The listing builds one solid part. Answer for the finished solid, in the listing's coordinates (mm). Face numbers are marked on the shaded views. A direction names the side the tool comes from. Coordinates: 2 decimals unless noted, no trailing zeros. Loops run counter-clockwise (first coordinate to the right, second up) from the corner with the lowest first, then second, coordinate; pieces in that order, holes last. Notation, with made-up numbers: (-24, -37) - (18, -37) arc R25 ccw to (18, -6) - close; hole circle Ø5 at (75.25, -13.5). An arc over 180 degrees is marked (long way). Return JSON: item names as keys, results as strings. Group by question number.
1. Each of these flat-tipped pins is pushed along its axis until it touches: P1, Ø8, axis at y = -22.5, z = 14.5, coming from the -X side; P2, Ø1, axis at y = -4.5, z = 14, coming from the +X side; P3, Ø5, axis at y = -8.5, z = 7, coming from the +X side. Where does it stop, or does it pass through?
2. Section C-C (y = -10) is taken. Write down the section's boundary in (x, z), and give its area (3 significant figures).
3. Section B-B (y = -2.5) is taken. Write down the section's boundary in (x, z), and give its area (3 significant figures).
4. Which of the six approach directions +Z, -Z, +X, -X, +Y, -Y give full straight-line access (tool end or side, diameter ignored) to the marked faces 1 and 2?
5. Find the intervals of material crossed by line 1 along X through (y, z) = (-16.5, -0.5); line 2 along X through (y, z) = (-2, 11.5); line 3 along X through (y, z) = (-13.75, 18), in increasing order.
6. The mould has two halves that part along X. Classify the marked faces 3, 4, 5 and 6: pulls with the +X half, pulls with the -X half, needs draft (parallel to the pull), parting line crosses it, or undercut.
7. Section A-A (y = -18) is taken. Write down the section's boundary in (x, z).
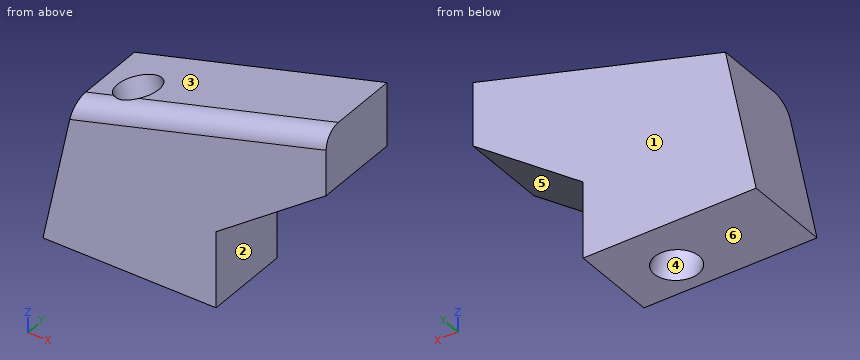
```python
from build123d import *

# Parameters (mm, degrees)
F1_DEPTH    = 25.4
F2_R        = 6.35
F3_DEPTH    = 62.0948563832
F4_T1_DEPTH = 102.4319350424


# Not quite as in the source:
# - a fillet or chamfer that OpenCascade refuses, or shapes differently, is made with other operations: its cross-section is extruded or revolved along the edge and cut away or added


with BuildPart() as f1:
    # F0 (on Front) → F1 (new body)
    with BuildSketch(Plane.XZ):
        Polygon((-12.7767093225, -11.5208044833), (-12.7767093225, 10.8061201186), (19.5394920482, 34.4463924892), (19.5394920482, 53.020893242), (-54.5708905419, 32.0073212298), (-63.5767093225, -11.5208044833), align=None)
    extrude(amount=F1_DEPTH)

    # F2 (on face) → F3 (cut, through all)
    with BuildSketch(Plane(origin=(-12.4610134404, 0, 43.9473342748), x_dir=(0.96207349, 0, 0.2727903953), z_dir=(-0.2727903953, 0, 0.96207349))):
        with Locations((-31.4930230379, -15.3000373393)):
            Circle(F2_R)
    extrude(amount=-F3_DEPTH, mode=Mode.SUBTRACT)

    # F4: fillet of radius 5.08 on 1 edges, made by hand

    # F4_s2 → F4_t1 (cut)
    with BuildSketch(Plane(origin=(44.218838812, 0, 12.5379969877), x_dir=(0, 1, 0), z_dir=(-0.96207349, 0, -0.2727903953))):
        with BuildLine():
            ThreePointArc((-25.4, -40.5998100459), (-23.9121024484, -44.1919124943), (-20.32, -45.6798100459))
            Line((-20.32, -45.6798100459), (-25.4, -45.6798100459))
            Line((-25.4, -45.6798100459), (-25.4, -40.5998100459))
        make_face()
    extrude(amount=F4_T1_DEPTH, mode=Mode.SUBTRACT)


solid = f1.part
```
The answers:
{
 "1": {"P1": "stops at x = -59.02", "P2": "stops at x = -7.73", "P3": "stops at x = -12.78"},
 "2": {"outline": "(-63.58, -11.52) - (-33.1, -11.52) - (-46.12, 34.4) - (-54.57, 32.01) - close; (-39.39, 36.31) - (-25.83, -11.52) - (-12.78, -11.52) - (-12.78, 10.81) - (19.54, 34.45) - (19.54, 53.02) - close", "area": "2,760 mm2"},
 "3": {"outline": "(-63.58, -11.52) - (-12.78, -11.52) - (-12.78, 10.81) - (19.54, 34.45) - (19.54, 53.02) - (-54.57, 32.01) - close", "area": "3,100 mm2"},
 "4": {"face 1": "+Z, -Z, +X, -X, +Y", "face 2": "-Z, +X, +Y, -Y"},
 "5": {"line 1": "x = -61.3 to -39.07, -26.11 to -12.78", "line 2": "x = -58.81 to -11.83", "line 3": "x = -57.47 to -44.24, -31.44 to -2.94"},
 "6": {"face 3": "pulls with the -X half", "face 4": "undercut", "face 5": "pulls with the +X half", "face 6": "needs draft"},
 "7": {"outline": "(-63.58, -11.52) - (-35.44, -11.52) - (-48.29, 33.79) - (-54.57, 32.01) - close; (-37.23, 36.92) - (-23.49, -11.52) - (-12.78, -11.52) - (-12.78, 10.81) - (19.54, 34.45) - (19.54, 53.02) - close"}
}
